Can you work these out from the model? Positions are in its coordinate system, mm. A direction names the side the tool comes from. Give positions to 0.01 mm unless a question says otherwise; leave off trailing zeros. Order: outer loops, then holes, each group sorted by start corner. A loop starts at its lowest first (then second) coordinate and runs counter-clockwise, first axis right, second up. Notation, with made-up numbers: (3.5, -9.5) - (38.5, -9.5) arc R11 ccw to (38.5, 6.5) - close; hole circle Ø9 at (-18, -13). An arc over 180 degrees is marked (long way). Answer as a JSON object with one key per item and string values.
```python
from build123d import *

# Parameters (mm, degrees)
SKETCH_1_W          = 54
SKETCH_1_H          = 50
EXTRUDE_1_DEPTH     = 24
SKETCH_2_R          = 1.55
CUT_EXTRUDE_1_DEPTH = 25
EXTRUDE_2_DEPTH     = 24
SKETCH_5_W          = 42
SKETCH_5_H          = 50
CUT_EXTRUDE_3_DEPTH = 20
CUT_EXTRUDE_4_DEPTH = 3
SKETCH_7_R          = 15
CUT_EXTRUDE_5_DEPTH = 25
SKETCH_11_R         = 20
SKETCH_11_R_2       = 15
EXTRUDE_3_DEPTH     = 7.5
SKETCH_12_R         = 21
SKETCH_12_R_2       = 20
EXTRUDE_4_DEPTH     = 0.5


with BuildPart() as part:
    # 草图1 → 凸台-拉伸1 (new body)
    with BuildSketch(Plane.XY):
        Rectangle(SKETCH_1_W, SKETCH_1_H)
    extrude(amount=EXTRUDE_1_DEPTH)

    # 草图2 → 切除-拉伸1 (cut, through all)
    with BuildSketch(Plane.XY.offset(24)):
        with Locations((-24, 15)):
            Circle(SKETCH_2_R)
        with Locations((24, 15)):
            Circle(SKETCH_2_R)
        with Locations((24, -19)):
            Circle(SKETCH_2_R)
        with Locations((-24, -19)):
            Circle(SKETCH_2_R)
    extrude(amount=-CUT_EXTRUDE_1_DEPTH, mode=Mode.SUBTRACT)

    # 草图3 → 凸台-拉伸2 (add)
    with BuildSketch(Plane.XY.offset(24)):
        with BuildLine():
            Line((-27, 25), (27, 25))
            ThreePointArc((27, 25), (0, 36.483329628), (-27, 25))
        make_face()
    extrude(amount=-EXTRUDE_2_DEPTH)

    # 草图5 → 切除-拉伸3 (cut)
    with BuildSketch(Plane.XY.offset(24)):
        Rectangle(SKETCH_5_W, SKETCH_5_H)
    extrude(amount=-CUT_EXTRUDE_3_DEPTH, mode=Mode.SUBTRACT)

    # 草图6 → 切除-拉伸4 (cut)
    with BuildSketch(Plane(origin=(0, 0, 0), x_dir=(-1, 0, 0), z_dir=(0, 0, -1))):
        with BuildLine():
            Line((-27, -16), (-24, -16))
            ThreePointArc((-24, -16), (-21, -19), (-24, -22))
            Line((-24, -22), (-27, -22))
            Line((-27, -22), (-27, -16))
        make_face()
        with BuildLine():
            Line((-27, 18), (-27, 12))
            Line((-27, 12), (-24, 12))
            ThreePointArc((-24, 12), (-21, 15), (-24, 18))
            Line((-24, 18), (-27, 18))
        make_face()
        with BuildLine():
            Line((27, -16), (24, -16))
            ThreePointArc((24, -16), (21, -19), (24, -22))
            Line((24, -22), (27, -22))
            Line((27, -22), (27, -16))
        make_face()
        with BuildLine():
            Line((27, 18), (24, 18))
            ThreePointArc((24, 18), (21, 15), (24, 12))
            Line((24, 12), (27, 12))
            Line((27, 12), (27, 18))
        make_face()
    extrude(amount=-CUT_EXTRUDE_4_DEPTH, mode=Mode.SUBTRACT)

    # 草图7 → 切除-拉伸5 (cut, through all)
    with BuildSketch(Plane(origin=(0, 0, 0), x_dir=(-1, 0, 0), z_dir=(0, 0, -1))):
        with Locations((0, -1)):
            Circle(SKETCH_7_R)
    extrude(amount=-CUT_EXTRUDE_5_DEPTH, mode=Mode.SUBTRACT)

    # 草图11 → 凸台-拉伸3 (add)
    with BuildSketch(Plane(origin=(0, 0, 0), x_dir=(-1, 0, 0), z_dir=(0, 0, -1))):
        with Locations((0, -1)):
            Circle(SKETCH_11_R)
        with Locations((0, -1)):
            Circle(SKETCH_11_R_2, mode=Mode.SUBTRACT)
    extrude(amount=EXTRUDE_3_DEPTH)

    # 草图12 → 凸台-拉伸4 (add)
    with BuildSketch(Plane(origin=(0, 0, 0), x_dir=(-1, 0, 0), z_dir=(0, 0, -1))):
        with Locations((0, -1)):
            Circle(SKETCH_12_R)
        with Locations((0, -1)):
            Circle(SKETCH_12_R_2, mode=Mode.SUBTRACT)
    extrude(amount=EXTRUDE_4_DEPTH)


solid = part.part
```
Q1. Which directions (+Z, -Z, +X, -X, +Y, -Y) give clear straight access to the entire face, cutting with the end or side of a thin tool? Please do faces 1 (the face through (-6, 20, 0)), 2 (the face through (-26, -16, 1)), 3 (the face through (-27, 0, 12)), 4 (the face through (21, -19, 1)).
Recorded:
{"face 1": "-Z", "face 2": "-Z, -X", "face 3": "+Z, -Z, -X, +Y, -Y", "face 4": "-Z, +X"}
Q2. I need wall thicknesses on L1, parallel to X at y = 18.5, z = 14; L2, parallel to Y at x = 0, z = 1.35; L3, parallel to Y at x = 24, z = 12. Which ranges of each line are inside material? Lowest first, please.
Recorded:
{"L1": "x = -27 to -21, 21 to 27", "L2": "y = -25 to -16, 14 to 36.48", "L3": "y = -25 to -20.55, -17.45 to 13.45, 16.55 to 27.79"}
Q3. If we section it at C-C, the plane z = 10.5: Please give me the cut outline in (x, y), then the cut area to 3 significant figures.
Recorded:
{"outline": "(-27, -25) - (-21, -25) - (-21, 25) - (21, 25) - (21, -25) - (27, -25) - (27, 25) arc R37.48 ccw to (-27, 25) - close; hole circle Ø3.1 at (-24, -19); hole circle Ø3.1 at (-24, 15); hole circle Ø3.1 at (24, -19); hole circle Ø3.1 at (24, 15)", "area": "998 mm^2"}
Q4. If we section it at B-B, the plane y = -1: Please give me the cut outline in (x, z), then the cut area to 3 significant figures.
Recorded:
{"outline": "(-27, 0) - (-21, 0) - (-21, -0.5) - (-20, -0.5) - (-20, -7.5) - (-15, -7.5) - (-15, 4) - (-21, 4) - (-21, 24) - (-27, 24) - close; (15, -7.5) - (20, -7.5) - (20, -0.5) - (21, -0.5) - (21, 0) - (27, 0) - (27, 24) - (21, 24) - (21, 4) - (15, 4) - close", "area": "412 mm^2"}
Q5. If we section it at D-D, the plane y = -19: Please give me the cut outline in (x, z), then the cut area to 3 significant figures.
Recorded:
{"outline": "(-27, 3) - (-25.55, 3) - (-25.55, 24) - (-27, 24) - close; (-22.45, 3) - (-21, 3) - (-21, 0) - (-10.82, 0) - (-10.82, -0.5) - (-8.72, -0.5) - (-8.72, -7.5) - (8.72, -7.5) - (8.72, -0.5) - (10.82, -0.5) - (10.82, 0) - (21, 0) - (21, 3) - (22.45, 3) - (22.45, 24) - (21, 24) - (21, 4) - (-21, 4) - (-21, 24) - (-22.45, 24) - close; (25.55, 3) - (27, 3) - (27, 24) - (25.55, 24) - close", "area": "423 mm^2"}
Q6. We'd pull the mould along Y, two halves only. Please class faces 5 (the face through (-25.3, 13.7, 3)), 6 (the face through (0, 25, 14)), 7 (the face through (25.4, 13.7, 3)), 8 (the face through (0, 26, 24)): released by +Y, released by -Y, zero draft, split by the parting line, or undercut.
Recorded:
{"face 5": "undercut", "face 6": "released by -Y", "face 7": "undercut", "face 8": "zero draft"}
Q7. If we section it at A-A, the plane x = 0: Please give me the cut outline in (y, z), then the cut area to 3 significant figures.
Recorded:
{"outline": "(-25, 0) - (-22, 0) - (-22, -0.5) - (-21, -0.5) - (-21, -7.5) - (-16, -7.5) - (-16, 4) - (-25, 4) - close; (14, -7.5) - (19, -7.5) - (19, -0.5) - (20, -0.5) - (20, 0) - (36.48, 0) - (36.48, 24) - (25, 24) - (25, 4) - (14, 4) - close", "area": "432 mm^2"}
Q8. I'm going to push flat-ended pins straight in: pin 1 Ø1.9 at (x, y) = (24, -19) entering from +Z; pin 2 Ø10 at (x, z) = (8.5, 20) entering from +Y; pin 3 Ø10 at (x, y) = (-12.5, 17) entering from +Z; pin 4 Ø6 at (x, z) = (-9, 12.5) entering from -Y. Where does each tip first touch, or does it pass through?
Recorded:
{"pin 1": "passes through", "pin 2": "stops at y = 36.32", "pin 3": "stops at z = 4", "pin 4": "stops at y = 25"}
